from build123d import *

# Parameters (mm, degrees)
SKETCH3_R           = 4.5
BOSS_EXTRUDE2_DEPTH = 2.5
BOSS_EXTRUDE3_DEPTH = 5
CIRPATTERN1_COUNT   = 8
SKETCH7_R           = 1.5
CUT_EXTRUDE1_DEPTH  = 5


with BuildPart() as part:
    # Sketch3 → Boss-Extrude2 (new body, symmetric)
    with BuildSketch(Plane(origin=(0, 0, 0), x_dir=(1, 0, 0), z_dir=(0, 1, 0))):
        with Locations((-6, -42.5)):
            Circle(SKETCH3_R)
    extrude(amount=BOSS_EXTRUDE2_DEPTH, both=True)

    # Sketch5 → Boss-Extrude3 (add, through all)
    with BuildSketch(Plane.XZ.offset(2.5)):
        with BuildLine():
            Line((-7.58091961, 46.713157152), (-4.460558472, 46.728489066))
            add(Edge.make_bspline(
                [(-7.58091961, 46.713157152), (-5.992864636, 53.279234709), (-4.460558472, 46.728489066)],
                knots=[0, 0, 0, 1, 1, 1], degree=2))
        make_face()
    boss_extrude3 = extrude(amount=-BOSS_EXTRUDE3_DEPTH)

    # CirPattern1: Boss-Extrude3 ×8 about axis
    cirpattern1_axis = Axis((-6, -2.5, 42.5), (0, 1, 0))
    for i in range(1, CIRPATTERN1_COUNT):
        add(boss_extrude3.rotate(cirpattern1_axis, i * 360 / CIRPATTERN1_COUNT))

    # Sketch7 → Cut-Extrude1 (cut)
    with BuildSketch(Plane.XZ.offset(2.5)):
        with Locations((-6, 42.5)):
            Circle(SKETCH7_R)
    extrude(amount=-CUT_EXTRUDE1_DEPTH, mode=Mode.SUBTRACT)


solid = part.part
For this review, take the finished solid that the model builds, in its own axes (mm). Round coordinates to 2 decimals unless told otherwise and drop trailing zeros. Use a Markdown table: item, result. Add a question column.
Item 1: Add section A-A, the plane z = 47.5. State how many separate pieces and enclosed holes the cut face has, then the cut area to 3 significant figures.
Item 2: To check wall thickness, follow line 1 along Z through (x, y) = (-6, -0.6); line 2 along X through (y, z) = (0.85, 47.5); line 3 along Z through (x, y) = (-6.5, -1.15). State the ranges of each line that lie inside material, in increasing order.
Item 3: Insertion check: pin 1 (2.5 mm diameter, centred on x = -6, z = 42.5, fed in from -Y). The pin has a flat end and moves straight along its axis. Give the tip position at first contact, or say it passes through.
Geometry results:
| question | item | result |
|---|---|---|
| 1 | separate pieces | 3 |
| 1 | enclosed holes | 0 |
| 1 | area | 32.7 mm² |
| 2 | line 1 | z = 35 to 41, 44 to 50 |
| 2 | line 2 | x = -11.43 to -9.54, -7.38 to -4.65, -2.5 to -0.57 |
| 2 | line 3 | z = 35.35 to 41.09, 43.91 to 49.67 |
| 3 | pin 1 | passes through |
